Check sheet for the modelled part. Datum: model origin and axes. Units: mm. A direction names the side the tool comes from. Round coordinates to 2 decimals unless told otherwise and drop trailing zeros. Order: outer loops, then holes, each group sorted by start corner. A loop starts at its lowest first (then second) coordinate and runs counter-clockwise, first axis right, second up.
Q1. Mould release check, pull along Z, two halves, no side actions. Record for faces 4 (the flat face through (0, 6, 0)), 5 (the flat face through (18.2, 94, 19)): +Z half, -Z half, draft (parallel to the pull), parting line (faces both ways), or undercut.
Q2. Cross-section at B-B on z = -2.5. Record the cut outline in (x, y), then the cut area to 3 significant figures.
Q3. Depth check by flat-ended pin: P1, Ø1.8, axis at y = 42.5, z = -20, coming from the +X side; P2, Ø2, axis at x = 12.5, y = 62.5, coming from the -Z side; P3, Ø5, axis at x = -14.5, z = -18, coming from the +Y side. Enter the tip coordinate at first touch or a pass-through.
Q4. Cross-section at C-C on y = 69.5. Record the cut outline in (x, z), then the cut area to 3 significant figures.
Q5. Cross-section at D-D on x = -23.5. Record the cut outline in (y, z), then the cut area to 3 significant figures.
Q6. Scan lines: probe 1 along X at (y, z) = (4.1, -2.5); probe 2 along Z at (x, y) = (-28.5, 34.5); probe 3 along X at (y, z) = (36.1, -17.8). Record each from-to range of solid material in increasing order.
Q7. Set-up check for faces 1 (the flat face through (38, 23.616, 19)), 2 (the flat face through (-13.8, 94, 19)), 3 (the flat face through (32, 3, 0)): record each of +Z, -Z, +X, -X, +Y, -Y from which the full face is reachable in a straight line by a thin tool's end or side.
Q8. Cross-section at A-A on z = -17. Record the cut outline in (x, y).
from build123d import *

# Parameters (mm, degrees)
CROQUIS1_W              = 64
CROQUIS1_H              = 43
CROQUIS1_R              = 2
SALIENTE_EXTRUIR1_DEPTH = 6
CROQUIS2_W              = 64
CROQUIS2_H              = 6
SALIENTE_EXTRUIR2_DEPTH = 99
CROQUIS3_R              = 2.3
CORTAR_EXTRUIR1_DEPTH   = 118.889779031
SALIENTE_EXTRUIR3_DEPTH = 6
CROQUIS5_W              = 64
CROQUIS5_H              = 6
SALIENTE_EXTRUIR4_DEPTH = 46
CORTAR_EXTRUIR2_START   = -6
CROQUIS6_R              = 2.3
CORTAR_EXTRUIR2_DEPTH   = 6
SALIENTE_EXTRUIR5_START = -6
SALIENTE_EXTRUIR5_DEPTH = 6


with BuildPart() as part:
    # Croquis1 → Saliente-Extruir1 (new body)
    with BuildSketch(Plane(origin=(0, 0, 0), x_dir=(1, 0, 0), z_dir=(0, 1, 0))):
        Rectangle(CROQUIS1_W, CROQUIS1_H)
        with Locations(Location((19.040268394, 2.5, 0), (0, 0, 270))):
            Circle(CROQUIS1_R, mode=Mode.SUBTRACT)
        with Locations(Location((-13.040268394, 2.5, 0), (0, 0, 90))):
            Circle(CROQUIS1_R, mode=Mode.SUBTRACT)
    extrude(amount=SALIENTE_EXTRUIR1_DEPTH)

    # Croquis2 → Saliente-Extruir2 (add)
    with BuildSketch(Plane(origin=(0, 6, 0), x_dir=(1, 0, 0), z_dir=(0, 1, 0))):
        with Locations((0, -18.5)):
            Rectangle(CROQUIS2_W, CROQUIS2_H)
    extrude(amount=SALIENTE_EXTRUIR2_DEPTH)

    # Croquis3 → Cortar-Extruir1 (cut, through all)
    with BuildSketch(Plane.XY.offset(21.5)):
        with Locations((3.7, 36.1)):
            Circle(CROQUIS3_R)
        with BuildLine():
            Line((-7.3, 75), (-7.3, 86))
            ThreePointArc((-7.3, 86), (3.7, 97), (14.7, 86))
            Line((14.7, 86), (14.7, 75))
            ThreePointArc((14.7, 75), (3.7, 64), (-7.3, 75))
        make_face()
        with BuildLine():
            Line((-13.8, 88), (-13.8, 100))
            ThreePointArc((-13.8, 100), (-12.3, 101.5), (-10.8, 100))
            Line((-10.8, 100), (-10.8, 88))
            ThreePointArc((-10.8, 88), (-12.3, 86.5), (-13.8, 88))
        make_face()
        with BuildLine():
            Line((-13.8, 73), (-13.8, 61))
            ThreePointArc((-13.8, 61), (-12.3, 59.5), (-10.8, 61))
            Line((-10.8, 61), (-10.8, 73))
            ThreePointArc((-10.8, 73), (-12.3, 74.5), (-13.8, 73))
        make_face()
        with BuildLine():
            Line((21.2, 88), (21.2, 100))
            ThreePointArc((21.2, 100), (19.7, 101.5), (18.2, 100))
            Line((18.2, 100), (18.2, 88))
            ThreePointArc((18.2, 88), (19.7, 86.5), (21.2, 88))
        make_face()
        with BuildLine():
            Line((21.2, 73), (21.2, 61))
            ThreePointArc((21.2, 61), (19.7, 59.5), (18.2, 61))
            Line((18.2, 61), (18.2, 73))
            ThreePointArc((18.2, 73), (19.7, 74.5), (21.2, 73))
        make_face()
    extrude(amount=-CORTAR_EXTRUIR1_DEPTH, mode=Mode.SUBTRACT)

    # Croquis4 → Saliente-Extruir3 (add)
    with BuildSketch(Plane.XY.offset(21.5)):
        with BuildLine():
            Line((32, 0), (42.927948292, 0))
            Line((42.927948292, 0), (42.927948292, 23.616164973))
            Line((42.927948292, 23.616164973), (32, 23.616164973))
            Line((32, 23.616164973), (32, 16.055291722))
            ThreePointArc((32, 16.055291722), (36.937550226, 15.5), (32, 14.944708278))
            Line((32, 14.944708278), (32, 0))
        make_face()
    extrude(amount=-SALIENTE_EXTRUIR3_DEPTH)

    # Croquis5 → Saliente-Extruir4 (add)
    with BuildSketch(Plane(origin=(0, 6, 0), x_dir=(1, 0, 0), z_dir=(0, 1, 0))):
        with Locations((0, 18.5)):
            Rectangle(CROQUIS5_W, CROQUIS5_H)
    extrude(amount=SALIENTE_EXTRUIR4_DEPTH)

    # Croquis6 → Cortar-Extruir2 (cut)
    with BuildSketch(Plane(origin=(0, 0, -21.5), x_dir=(-1, 0, 0), z_dir=(0, 0, -1)).offset(CORTAR_EXTRUIR2_START)):
        with Locations(Location((-3.7, 36.1, 0), (0, 0, 180))):
            Circle(CROQUIS6_R)
    extrude(amount=CORTAR_EXTRUIR2_DEPTH, mode=Mode.SUBTRACT)

    # Croquis7 → Saliente-Extruir5 (add)
    with BuildSketch(Plane(origin=(0, 0, -21.5), x_dir=(-1, 0, 0), z_dir=(0, 0, -1)).offset(SALIENTE_EXTRUIR5_START)):
        with BuildLine():
            Line((-32, 23.616164973), (-42.927948292, 23.616164973))
            Line((-42.927948292, 23.616164973), (-42.927948292, 0))
            Line((-42.927948292, 0), (-32, 0))
            Line((-32, 0), (-32, 14.944708278))
            ThreePointArc((-32, 14.944708278), (-36.937550226, 15.5), (-32, 16.055291722))
            Line((-32, 16.055291722), (-32, 23.616164973))
        make_face()
    extrude(amount=SALIENTE_EXTRUIR5_DEPTH)


solid = part.part
Results found:
1. face 4: undercut
1. face 5: draft
2. outline: (-32, 0) - (-15.04, 0) - (-15.04, 6) - (-32, 6) - close; (-11.04, 0) - (17.04, 0) - (17.04, 6) - (-11.04, 6) - close; (21.04, 0) - (32, 0) - (32, 6) - (21.04, 6) - close
2. area: 336 mm2
3. P1: stops at x = 32
3. P2: stops at z = 15.5
3. P3: stops at y = 52
4. outline: (-32, 15.5) - (-13.8, 15.5) - (-13.8, 21.5) - (-32, 21.5) - close; (-10.8, 15.5) - (-5.83, 15.5) - (-5.83, 21.5) - (-10.8, 21.5) - close; (13.23, 15.5) - (18.2, 15.5) - (18.2, 21.5) - (13.23, 21.5) - close; (21.2, 15.5) - (32, 15.5) - (32, 21.5) - (21.2, 21.5) - close
4. area: 234 mm2
5. outline: (0, -21.5) - (52, -21.5) - (52, -15.5) - (6, -15.5) - (6, 15.5) - (105, 15.5) - (105, 21.5) - (0, 21.5) - close
5. area: 1,130 mm2
6. probe 1: x = -32 to -15.04, -11.04 to 17.04, 21.04 to 32
6. probe 2: z = -21.5 to -15.5, 15.5 to 21.5
6. probe 3: x = -32 to 1.4, 6 to 32
7. face 1: +Z, -Z, +X, +Y
7. face 2: +Z, -Z
7. face 3: +X, +Y, -Y
8. outline: (-32, 0) - (42.93, 0) - (42.93, 23.62) - (32, 23.62) - (32, 52) - (-32, 52) - close; hole circle Ø4.6 at (3.7, 36.1); hole (32, 14.94) arc R2.5 ccw (long way) to (32, 16.06) - close
